Autodesk Inventor part; units mm, degrees
ref_plane "YZ Plane" through (0, 0, 0) normal (1, 0, 0) x (0, 1, 0)
ref_plane "XZ Plane" through (0, 0, 0) normal (0, 1, 0) x (-1, 0, 0)
ref_plane "XY Plane" through (0, 0, 0) normal (0, 0, 1) x (1, 0, 0)
sketch "Sketch1" plane through (0, 0, 0) normal (0, 0, 1) x (1, 0, 0)
  circle A0 centre (0, 0) radius 11
  circle A1 centre (0, 0) radius 15.6205
  line L0 (26, 8) -> (11, 8)
  line L1 (11, 8) -> (11, -8)
  line L2 (11, -8) -> (26, -8)
  line L3 (26, -8) -> (26, 8)
  line L4 (-65.7, 10) -> (-12, 10)
  line L5 (-12, 10) -> (-12, -10)
  line L6 (-12, -10) -> (-65.7, -10)
  line L7 (-65.7, -10) -> (-65.7, 10)
  point P0 (13.4164, 8)
  point P1 (13.4164, -8)
  point P2 (-12, -10)
  point P3 (-12, 10)
  point P4 (-12, 0)
  dimension "d0" = 22
  dimension "d1" = 31.241
  dimension "d10" = 15
  dimension "d11" = 16
  dimension "d45" = 53.7
  dimension "d46" = 20
extrude "Extrusion1" add sketch "Sketch1" along normal blind 14.7
sketch "Sketch2" plane through (0, 0, 14.7) normal (0, 0, 1) x (1, 0, 0)
  circle A0 centre (0, 0) radius 11
  line L0 (26, -8) -> (26, 8)
  line L1 (26, 0) -> (10.8, 0)
  line L2 (10.8, 0) -> (10.8, 1)
  line L3 (10.8, 1) -> (26, 1)
  line L4 (26, 1) -> (26, 0)
  line L5 (26, 0) -> (10.8, 0)
  line L6 (10.8, 0) -> (10.8, -1)
  line L7 (10.8, -1) -> (26, -1)
  line L8 (26, -1) -> (26, 0)
  point P0 (10.9545, 1)
  point P1 (10.9545, -1)
  dimension "d20" = 15.2
  dimension "d21" = 1
  dimension "d22" = 1
extrude "Extrusion2" cut sketch "Sketch2" against normal blind 15 contours L1 L2 L3 A0 | L1 L0 L7 A0 | A0 L3 L0 L1 | A0 L7 L6 L1
sketch "Sketch3" plane through (13.4164, -8, 0) normal (0, -1, 0) x (1, 0, 0)
  line L0 (0, 0) -> (0, 14.7)
  line L1 (0, 0) -> (6.6555, 0)
  line L2 (6.6555, 0) -> (6.6555, 7.5)
  line L3 (6.6555, 7.5) -> (0, 7.5)
  line L4 (0, 7.5) -> (0, 0)
  point P0 (-13.4164, 0)
  dimension "d25" = 6.6555
  dimension "d26" = 7.5
hole "Hole1" at (20.0719, -8, 7.5) direction (0, 1, 0) diameter 4.5 depth 12.5 counterbore diameter 8.5 counterbore depth 3.5
sketch "Sketch4" plane through (13.4164, 8, 0) normal (0, 1, 0) x (1, 0, 0)
  line L0 (12.5836, 0) -> (0, 0)
  line L1 (0, 0) -> (6.6555, 0)
  line L2 (6.6555, 0) -> (6.6555, -7.5)
  line L3 (6.6555, -7.5) -> (0, -7.5)
  line L4 (0, -7.5) -> (0, 0)
  line L5 (6.6555, -7.5) -> (6.6555, -12)
  line L6 (6.6555, -7.5) -> (11.1555, -7.5) construction
  line L7 (6.6555, -12) -> (2.7584, -9.75)
  line L8 (2.7584, -9.75) -> (2.7584, -5.25)
  line L9 (2.7584, -5.25) -> (6.6555, -3)
  line L10 (6.6555, -3) -> (10.5526, -5.25)
  line L11 (10.5526, -5.25) -> (10.5526, -9.75)
  line L12 (10.5526, -9.75) -> (6.6555, -12)
  point P0 (-13.4164, 0)
  dimension "d51" = 6.6555
  dimension "d52" = 7.5
  dimension "d53" = 4.5
  dimension "d54" = 90
extrude "Extrusion3" cut sketch "Sketch4" against normal blind 4.2 contours L10 L11 L12 L5 L2 | L2 L3 L8 L9 | L5 L7 L8 L3
fillet "Fillet1" radius 2 2 edges at (-38.85, 10, 14.7) (-38.85, -10, 14.7)
fillet "Fillet2" radius 2 4 edges at (-12, -10, 6.35) (-12.4535, -9.4292, 14.0991) (-12, 10, 6.35) (-12.4535, 9.4292, 14.0991)
fillet "Fillet3" radius 2 2 edges at (26, -8, 7.35) (26, 8, 7.35)
properties part number "Clasp"
Verification items for the finished model (mm, model axes). A direction names the side the tool comes from. Coordinates: 2 decimals unless noted, no trailing zeros. Order: outer loops, then holes, each group sorted by start corner. A loop starts at its lowest first (then second) coordinate and runs counter-clockwise, first axis right, second up. Notation, with made-up numbers: (20.5, 0) -> (66.5, 0) arc R34 ccw to (66.5, 34) -> close; hole circle Ø6 at (71.5, -12.5). An arc over 180 degrees is marked (long way). Put each result on its own line as item: value. Start each with the question number.
1) Cross-section at A-A (x = 0). Enter the section's corners in (y, z).
2) Material ranges on L1, parallel to Y at x = 0, z = 10.75; L2, parallel to X at y = 2.3, z = 7.5; L3, parallel to X at y = -2.65, z = 7.5, recorded low to high.
3) Release check for a two-part mould opening along Z. For faces 6 (the cylindrical face through (15.858, -6.226, 8.053)), 7 (the flat face through (-20, 0, 0)), 8 (the flat face through (22, -4.5, 6)), 9 (the flat face through (-65.7, 0, 7)) record: pulls with the +Z half, pulls with the -Z half, needs draft (parallel to the pull), parting line crosses it, or undercut.
4) Cross-section at C-C (y = 0). Enter the section's corners in (x, z).
5) Cross-section at D-D (x = -41). Enter the section's corners in (y, z).
6) Go/stop test with flat-tipped pins: pin 1 (8.5 mm diameter, centred on x = 17.5, z = 5.5, fed in from -Y); pin 2 (7 mm diameter, centred on x = 20.07, z = 7.5, fed in from +Y); pin 3 (1.5 mm diameter, centred on x = -22.5, z = 12.5, fed in from -Y); pin 4 (12 mm diameter, centred on x = 7, y = 4.5, fed in from +Z). Record where each tip stops, or that it passes through.
7) Cross-section at B-B (z = 1.25). Enter the section's corners in (x, y).
8) Tool access check on faces 1 (the flat face through (15, -8, 7)), 2 (the flat face through (-40, 10, 6)), 3 (the flat face through (15, 8, 7)), 4 (the flat face through (17, 1, 7)), 5 (the flat face through (21.993, 5.929, 4.109)). Record the directions out of +Z, -Z, +X, -X, +Y, -Y that give a thin tool (end or side, any length) a straight path to the whole face; none if there is none.
Geometry check:
1. outline: (-15.62, 0) -> (-11, 0) -> (-11, 14.7) -> (-15.62, 14.7) -> close; (11, 0) -> (15.62, 0) -> (15.62, 14.7) -> (11, 14.7) -> close
2. L1: y = -15.62 to -11, 11 to 15.62
2. L2: x = -65.7 to -10.76, 10.76 to 17.82, 22.32 to 26
2. L3: x = -65.7 to -10.68, 10.68 to 17.82, 22.32 to 26
3. face 6: undercut
3. face 7: pulls with the -Z half
3. face 8: undercut
3. face 9: needs draft
4. outline: (-65.7, 0) -> (-11, 0) -> (-11, 14.7) -> (-65.7, 14.7) -> close
5. outline: (-10, 0) -> (10, 0) -> (10, 12.7) arc R2 ccw to (8, 14.7) -> (-8, 14.7) arc R2 ccw to (-10, 12.7) -> close
6. pin 1: stops at y = -8.27
6. pin 2: stops at y = 3.8
6. pin 3: stops at y = -10
6. pin 4: stops at z = 14.7
7. outline: (-65.7, -10) -> (-12.9, -10) arc R2 cw to (-11.44, -10.64) arc R15.62 ccw to (13.42, -8) -> (24, -8) arc R2 ccw to (26, -6) -> (26, -1) -> (10.95, -1) arc R11 cw (long way) to (10.95, 1) -> (26, 1) -> (26, 6) arc R2 ccw to (24, 8) -> (13.42, 8) arc R15.62 ccw to (-11.44, 10.64) arc R2 cw to (-12.9, 10) -> (-65.7, 10) -> close
8. face 1: +Z, -Z, +X, -Y
8. face 2: +Z, -Z, -X, +Y
8. face 3: +Z, -Z, +X, +Y
8. face 4: +Z, -Z, +X
8. face 5: +Y
